Source: three-view drawing plus pictorial views. Frame: mm from the lowest corner of the part. A direction names the side the tool comes from. Round coordinates to 2 decimals unless told otherwise and drop trailing zeros. Write each loop counter-clockwise with the first axis right and the second up, starting at its lowest first coordinate (ties: lowest second). Pieces come first, ordered by that corner, then holes. Notation, with made-up numbers: (-23.75, -10.5) -> (21.25, -10.5) arc R17 cw to (21.25, 0.5) -> close; hole circle Ø2 at (48, 20.5). An arc over 180 degrees is marked (long way). Put each result on its own line as item: value.
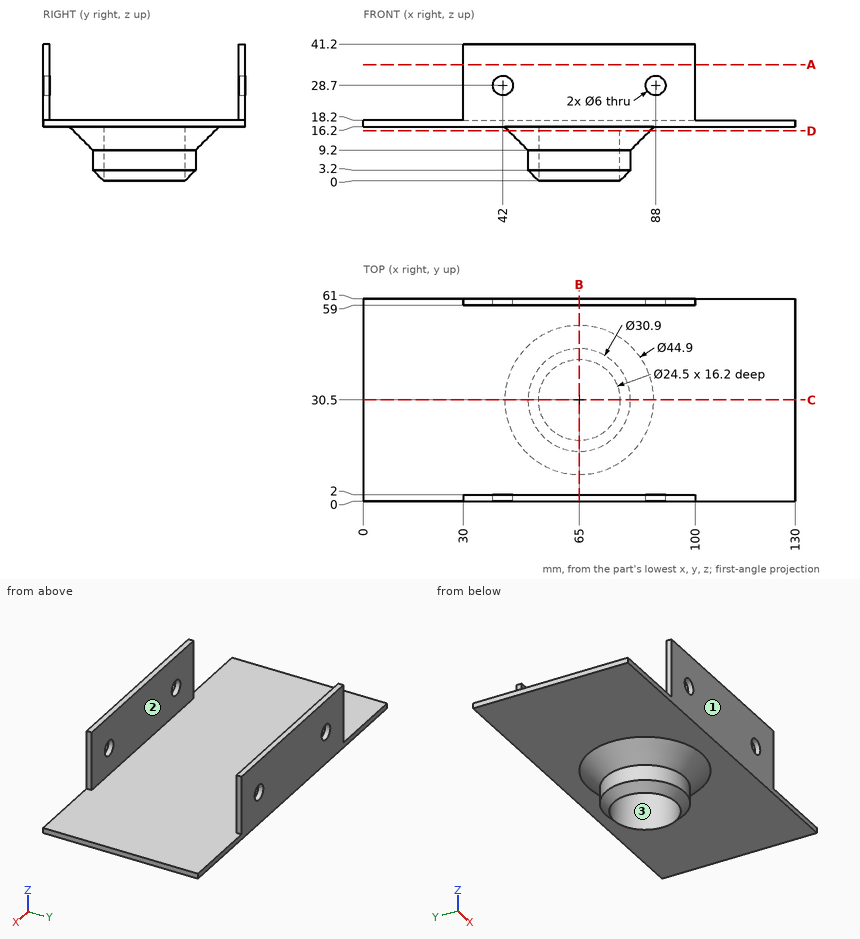
Q1. Cut plane B-B on x = 65. Output: boundary loops of the cut face in (y, z), and give its area (3 significant figures).
Ans:
outline: (0, 16.2) -> (8.05, 16.2) -> (15.05, 9.2) -> (15.05, 3.2) -> (18.25, 0) -> (18.25, 16.2) -> (42.75, 16.2) -> (42.75, 0) -> (45.95, 3.2) -> (45.95, 9.2) -> (52.95, 16.2) -> (61, 16.2) -> (61, 41.2) -> (59, 41.2) -> (59, 18.2) -> (2, 18.2) -> (2, 41.2) -> (0, 41.2) -> close
area: 356 mm^2
Q2. Cut plane C-C on y = 30.5. Output: boundary loops of the cut face in (x, z).
Ans:
outline: (0, 16.2) -> (42.55, 16.2) -> (49.55, 9.2) -> (49.55, 3.2) -> (52.75, 0) -> (52.75, 16.2) -> (77.25, 16.2) -> (77.25, 0) -> (80.45, 3.2) -> (80.45, 9.2) -> (87.45, 16.2) -> (130, 16.2) -> (130, 18.2) -> (0, 18.2) -> close
Q3. Material intervals for line 1 (Y direction, x = 74.5, z = 36.5); line 2 (Z direction, x = 42, y = 60.3); line 3 (X direction, y = 1, z = 28), sorted ascending. Write a range as [from, to].
Ans:
line 1: y = [0, 2], [59, 61]
line 2: z = [16.2, 25.7], [31.7, 41.2]
line 3: x = [30, 39.08], [44.92, 85.08], [90.92, 100]
Q4. Cut plane D-D on z = 15. Output: boundary loops of the cut face in (x, y).
Ans:
outline: circle Ø42.5 at (65, 30.5); hole circle Ø24.5 at (65, 30.5)
Q5. Cut plane A-A on z = 35. Output: boundary loops of the cut face in (x, y), and give its area (3 significant figures).
Ans:
outline: (30, 0) -> (100, 0) -> (100, 2) -> (30, 2) -> close; (30, 59) -> (100, 59) -> (100, 61) -> (30, 61) -> close
area: 280 mm^2
Q6. Pin query (flat end, axial travel): pin 1 (3.5 mm diameter, centred on x = 88, z = 28.7, fed in from -Y); pin 2 (1.6 mm diameter, centred on y = 60.5, z = 29.5, fed in from -X); pin 3 (4 mm diameter, centred on x = 69, y = 44.5, fed in from +Z); pin 4 (1 mm diameter, centred on y = 0.5, z = 26, fed in from +X). Return the tip coordinate at first contact, or that it passes through.
Ans:
pin 1: passes through
pin 2: stops at x = 30
pin 3: stops at z = 18.2
pin 4: stops at x = 100
Q7. Reachability of the marked faces 1, 2 and 3 from +Z, -Z, +X, -X, +Y, -Y: full face, straight path, thin tool, end or side. Return the list, or none.
Ans:
face 1: +Z, -Z, +X, -X, -Y
face 2: +Z, +X, -X
face 3: -Z
